Check sheet for the modelled part. Datum: model origin and axes. Units: mm. Coordinates: 2 decimals unless noted, no trailing zeros. Loops run counter-clockwise (first coordinate to the right, second up) from the corner with the lowest first, then second, coordinate; pieces in that order, holes last. Notation, with made-up numbers: M -1,74.25 L 8,74.25 A29 cw 8,111.25 Z; hole C 61.5,62 d1. An arc over 180 degrees is marked long. Use CSV: the item, a comma, the result in double quotes. Start each with the question number.
(1) Draft check along X on faces 1 (the cylindrical face through (-0.53, 1.01, -0.06)), 2 (the flat face through (-20, 1, 0)), 3 (the flat face through (0, 1, 5)). Enter one of: pulls with the +X half, pulls with the -X half, needs draft (parallel to the pull), parting line crosses it, or undercut.
(2) Scan lines: line 1 (X direction, y = 0.95, z = 1); line 2 (X direction, y = 0.45, z = -0.75); line 3 (X direction, y = 1.65, z = -1.75). Record each from-to range of solid material in increasing order.
(3) Section check A-A on y = 0.8. Record the cut outline in (x, z), and give its area (3 significant figures).
(4) Section check D-D on x = 5.5. Record the cut outline in (y, z).
(5) Section check B-B on x = -12. Record the cut outline in (y, z), and give its area (3 significant figures).
(6) Go/stop test with flat-tipped pins: pin 1 Ø2.5 at (x, z) = (0.77, 0) entering from -Y; pin 2 Ø3.5 at (x, z) = (-12.78, 0) entering from +Y. Record where each tip stops, or that it passes through.
(7) Section check C-C on z = 0.75. Record the cut outline in (x, y), and give its area (3 significant figures).
from build123d import *

# Parameters (mm, degrees)
SKETCH1_W                = 40
SKETCH1_H                = 10
BOSS_EXTRUDE1_DEPTH      = 2
SKETCH2_R                = 2.472864358
SKETCH2_R_2              = 1.3
CUT_EXTRUDE1_DEPTH       = 3
FILLET1_R                = 3
F_3_0_3_DIAMETER_HOLE1_D = 3


with BuildPart() as part:
    # Sketch1 → Boss-Extrude1 (new body)
    with BuildSketch(Plane(origin=(0, 0, 0), x_dir=(1, 0, 0), z_dir=(0, 1, 0))):
        Rectangle(SKETCH1_W, SKETCH1_H)
    extrude(amount=BOSS_EXTRUDE1_DEPTH)

    # Sketch2 → Cut-Extrude1 (cut)
    with BuildSketch(Plane(origin=(0, 2, 0), x_dir=(1, 0, 0), z_dir=(0, 1, 0))):
        with Locations((7.219918586, 0)):
            Circle(SKETCH2_R)
        with Locations((13.669918586, 0)):
            Circle(SKETCH2_R_2)
        with Locations((0.769918586, 0)):
            Circle(SKETCH2_R_2)
    extrude(amount=-CUT_EXTRUDE1_DEPTH, mode=Mode.SUBTRACT)

    # Fillet1
    fillet1_edges = [part.edges().sort_by_distance(p)[0] for p in [
        (20, 1, 5),
        (-20, 1, 5),
        (-20, 1, -5),
        (20, 1, -5),
    ]]
    fillet(fillet1_edges, radius=FILLET1_R)

    # Ø3.0 (3) Diameter Hole1 (through all)
    with Locations(Plane(origin=(0, 2, 0), x_dir=(1, 0, 0), z_dir=(0, 1, 0))):
        with Locations((-12.780081414, 0)):
            Hole(F_3_0_3_DIAMETER_HOLE1_D / 2)


solid = part.part
Outcome:
1,face 1,"undercut"
1,face 2,"pulls with the -X half"
1,face 3,"needs draft"
2,line 1,"x = -20 to -13.9, -11.66 to -0.06, 1.6 to 4.96, 9.48 to 12.84, 14.5 to 20"
2,line 2,"x = -20 to -14.08, -11.48 to -0.29, 1.83 to 4.86, 9.58 to 12.61, 14.73 to 20"
2,line 3,"x = -20 to 5.47, 8.97 to 20"
3,outline,"M -20,-2 A3 ccw -17,-5 L 17,-5 A3 ccw 20,-2 L 20,2 A3 ccw 17,5 L -17,5 A3 ccw -20,2 Z; hole C -12.78,0 d3; hole C 0.77,0 d2.6; hole C 7.22,0 d4.95; hole C 13.67,0 d2.6"
3,area,"355 mm²"
4,outline,"M 0,-5 L 2,-5 L 2,-1.78 L 0,-1.78 Z; M 0,1.78 L 2,1.78 L 2,5 L 0,5 Z"
5,outline,"M 0,-5 L 2,-5 L 2,-1.28 L 0,-1.28 Z; M 0,1.28 L 2,1.28 L 2,5 L 0,5 Z"
5,area,"14.9 mm²"
6,pin 1,"passes through"
6,pin 2,"stops at y = 2"
7,outline,"M -20,0 L -14.08,0 L -14.08,2 L -20,2 Z; M -11.48,0 L -0.29,0 L -0.29,2 L -11.48,2 Z; M 1.83,0 L 4.86,0 L 4.86,2 L 1.83,2 Z; M 9.58,0 L 12.61,0 L 12.61,2 L 9.58,2 Z; M 14.73,0 L 20,0 L 20,2 L 14.73,2 Z"
7,area,"56.9 mm²"
